Source: CAD feature listing. Evaluate the final solid. Frame: model axes, mm. A direction names the side the tool comes from. Give positions to 0.01 mm unless a question says otherwise; leave off trailing zeros. Write each loop counter-clockwise with the first axis right and the second up, starting at its lowest first coordinate (ties: lowest second). Pieces come first, ordered by that corner, then holes. Notation, with made-up numbers: (81, 45) -> (94, 45) arc R32 cw to (94, 73) -> close; hole circle Ø2 at (-23, 86). An arc over 180 degrees is marked (long way). Use one line per item in the form item = value. Start each with the question number.
(1) Draft query along X for faces 1 (the face through (5, -6, -20)), 2 (the face through (-25, -6, 0)), 3 (the face through (10.277, -6.084, -8.802)). Return one class per face: pulls with the +X half, pulls with the -X half, needs draft (parallel to the pull), parting line crosses it, or undercut.
(2) Cut plane B-B, the plane z = 27.5. Output: boundary loops of the cut face in (x, y).
(3) Cut plane A-A, the plane y = -6. Count the separate pieces of the cut face and the enclosed holes in it, and give its area (3 significant figures).
(4) Cut plane D-D, the plane x = 16. Output: boundary loops of the cut face in (y, z).
(5) First-contact query: P1, Ø4, axis at x = -12.5, y = -9, coming from the +Z side; P2, Ø1.5, axis at x = 8.5, y = -6.5, coming from the +Z side; P3, Ø6, axis at y = -8, z = 26.5, coming from the +X side. Flat tips, straight axial feed; report the tip coordinate or a pass-through.
(6) Cut plane C-C, the plane y = -10. Output: boundary loops of the cut face in (x, z).
(7) Material intervals for line 1 along X through (y, z) = (-8.5, -7); line 2 along Z through (x, y) = (-22.45, -6); line 3 along Z through (x, y) = (-21.3, -6), sorted ascending. Write a range as from..to.
(8) Set-up query: faces 4 (the face through (-15, -6, -33)), 5 (the face through (-16.972, -3.693, -31.936)), 6 (the face through (-12, -6, 20)), 7 (the face through (5, -6, 5)), 8 (the face through (-6, -12, 0)). Return all of +Z, -Z, +X, -X, +Y, -Y with unobstructed straight access to the full face (end or side cutting, diameter ignored); none if empty.
from build123d import *

# Parameters (mm, degrees)
F0_W      = 10
F0_H      = 15
F0_H_2    = 40
F1_DEPTH  = 12
F2_R      = 3
F3_DEPTH  = 10.001
F4_R      = 5
F4_R_2    = 3
F5_DEPTH  = 4
F6_R      = 3
F7_DEPTH  = 10.001
F8_R      = 5
F8_R_2    = 3
F9_DEPTH  = 4
F11_DEPTH = 12.001


with BuildPart() as f1:
    # F0 (on Front) → F1 (new body)
    with BuildSketch(Plane.XZ):
        with Locations((-20, 27.5)):
            Rectangle(F0_W, F0_H)
        with Locations((-20, 0)):
            Rectangle(F0_W, F0_H_2)
        with Locations((-20, -27.5)):
            Rectangle(F0_W, F0_H)
        with BuildLine():
            Line((-15, -20), (25, -20))
            Line((25, -20), (25, 20))
            Line((25, 20), (20, 20))
            ThreePointArc((20, 20), (5, 5), (-10, 20))
            Line((-10, 20), (-15, 20))
            Line((-15, 20), (-15, -20))
        make_face()
    extrude(amount=F1_DEPTH)

    # F2 (on face) → F3 (cut, through all)
    with BuildSketch(Plane.YZ.offset(-15)):
        with Locations((-6, 27.5)):
            Circle(F2_R)
    extrude(amount=-F3_DEPTH, mode=Mode.SUBTRACT)

    # F4 (on face) → F5 (cut)
    with BuildSketch(Plane.YZ.offset(-15)):
        with Locations((-6, 27.5)):
            Circle(F4_R)
        with Locations((-6, 27.5)):
            Circle(F4_R_2, mode=Mode.SUBTRACT)
    extrude(amount=-F5_DEPTH, mode=Mode.SUBTRACT)

    # F6 (on face) → F7 (cut, through all)
    with BuildSketch(Plane.YZ.offset(-15)):
        with Locations((-6, -27.5)):
            Circle(F6_R)
    extrude(amount=-F7_DEPTH, mode=Mode.SUBTRACT)

    # F8 (on face) → F9 (cut)
    with BuildSketch(Plane.YZ.offset(-15)):
        with Locations((-6, -27.5)):
            Circle(F8_R)
        with Locations((-6, -27.5)):
            Circle(F8_R_2, mode=Mode.SUBTRACT)
    extrude(amount=-F9_DEPTH, mode=Mode.SUBTRACT)

    # F10 (on face) → F11 (cut, through all)
    with BuildSketch(Plane.XZ.offset(12)):
        with BuildLine():
            Line((-22, -7), (-10, -7))
            ThreePointArc((-10, -7), (-16, -1), (-22, -7))
        make_face()
        with BuildLine():
            ThreePointArc((-22, -7), (-16, -13), (-10, -7))
            Line((-10, -7), (-22, -7))
        make_face()
        with BuildLine():
            Line((-6, -7), (6, -7))
            ThreePointArc((6, -7), (0, -1), (-6, -7))
        make_face()
        with BuildLine():
            ThreePointArc((-6, -7), (0, -13), (6, -7))
            Line((6, -7), (-6, -7))
        make_face()
        with BuildLine():
            Line((10, -7), (22, -7))
            ThreePointArc((22, -7), (16, -1), (10, -7))
        make_face()
        with BuildLine():
            ThreePointArc((10, -7), (16, -13), (22, -7))
            Line((22, -7), (10, -7))
        make_face()
    extrude(amount=-F11_DEPTH, mode=Mode.SUBTRACT)


solid = f1.part
Geometry says:
q1.face_1 = needs draft
q1.face_2 = pulls with the -X half
q1.face_3 = undercut
q2.outline = (-25, -12) -> (-15, -12) -> (-15, -11) -> (-19, -11) -> (-19, -9) -> (-25, -9) -> close; (-25, -3) -> (-19, -3) -> (-19, -1) -> (-15, -1) -> (-15, 0) -> (-25, 0) -> close
q3.separate_pieces = 3
q3.enclosed_holes = 3
q3.area = 1,460 mm^2
q4.outline = (-12, -20) -> (0, -20) -> (0, -13) -> (-12, -13) -> close; (-12, -1) -> (0, -1) -> (0, 9.8) -> (-12, 9.8) -> close
q5.P1 = 20
q5.P2 = 5.61
q5.P3 = -15
q6.outline = (-25, -35) -> (-15, -35) -> (-15, -30.5) -> (-19, -30.5) -> (-19, -24.5) -> (-15, -24.5) -> (-15, -20) -> (25, -20) -> (25, 20) -> (20, 20) arc R15 cw to (-10, 20) -> (-15, 20) -> (-15, 24.5) -> (-19, 24.5) -> (-19, 30.5) -> (-15, 30.5) -> (-15, 35) -> (-25, 35) -> close; hole circle Ø12 at (-16, -7); hole circle Ø12 at (0, -7); hole circle Ø12 at (16, -7)
q7.line_1 = -25..-22, -10..-6, 6..10, 22..25
q7.line_2 = -35..-30.5, -24.5..24.5, 30.5..35
q7.line_3 = -35..-30.5, -24.5..-9.81, -4.19..24.5, 30.5..35
q8.face_4 = -Z, +X, +Y, -Y
q8.face_5 = +X
q8.face_6 = +Z, +X, +Y, -Y
q8.face_7 = +Z, +Y, -Y
q8.face_8 = +Z, -Z, +X, -X, -Y
